Autodesk Inventor part; units mm, degrees
ref_plane "YZ Plane" through (0, 0, 0) normal (1, 0, 0) x (0, 1, 0)
ref_plane "XZ Plane" through (0, 0, 0) normal (0, 1, 0) x (-1, 0, 0)
ref_plane "XY Plane" through (0, 0, 0) normal (0, 0, 1) x (1, 0, 0)
sketch "Sketch1" plane through (0, 0, 0) normal (0, 1, 0) x (-1, 0, 0)
  line L0 (0, 0) -> (111.125, 0)
  line L1 (111.125, 0) -> (111.125, -88.9)
  line L2 (111.125, -88.9) -> (0, -88.9)
  line L3 (0, -88.9) -> (0, 0)
  dimension "d0" = 111.125
  dimension "d1" = 88.9
extrude "Extrusion1" add sketch "Sketch1" along normal blind 25.4
sketch "Sketch2" plane through (0, 25.4, 0) normal (0, 1, 0) x (1, 0, 0)
  line L0 (0, 88.9) -> (-111.125, 88.9)
  line L1 (-111.125, 0) -> (0, 0)
  line L2 (-27.305, 88.9) -> (-81.915, 88.9)
  line L3 (-81.915, 88.9) -> (-81.915, 0)
  line L4 (-81.915, 0) -> (-27.305, 0)
  line L5 (-27.305, 0) -> (-27.305, 88.9)
  line L6 (0, 0) -> (0, 88.9)
  dimension "d4" = 111.125
  dimension "d5" = 54.61
  dimension "d6" = 27.305
extrude "Extrusion2" cut sketch "Sketch2" against normal blind 3.175 contours L5 L1 L3 L0
sketch "Sketch4" plane through (-111.125, 0, 0) normal (0, 0, 1) x (1, 0, 0)
  line L0 (0, 0) -> (0, 25.4)
  line L1 (0, 19.05) -> (21.59, 25.4)
  line L2 (0, 25.4) -> (29.21, 25.4)
  point P0 (111.125, 0)
  dimension "d17" = 6.35
  dimension "d18" = 7.62
extrude "Extrusion4" cut sketch "Sketch4" against normal through all
fillet "Fillet2" radius 3.175 2 edges at (-111.125, 0, -44.45) (0, 25.4, -44.45)
properties part number "lift holder" material "PC/ABS Plastic"
Geometry check sheet. Reference: the model listing, model coordinates, mm. A direction names the side the tool comes from. Round coordinates to 2 decimals unless told otherwise and drop trailing zeros. Order: outer loops, then holes, each group sorted by start corner. A loop starts at its lowest first (then second) coordinate and runs counter-clockwise, first axis right, second up. Notation, with made-up numbers: M 16,82 L 66,82 A14 ccw 66,94 Z; hole C 13,63 d7. An arc over 180 degrees is marked long. Answer in a Markdown table with one row per item.
(1) Sectioned sample at A-A, the plane z = -17. Record the cut outline in (x, y) (3 decimals).
Responses:
| item | result |
|---|---|
| outline | M -111.125,3.175 A3.175 ccw -107.95,0 L 0,0 L 0,22.225 A3.175 ccw -3.175,25.4 L -27.305,25.4 L -27.305,22.225 L -81.915,22.225 L -81.915,25.4 L -89.535,25.4 L -111.125,19.05 Z |
(2) Go/stop test with flat-tipped pins: P1, Ø10, axis at x = -67, y = 8.5, coming from the +Z side; P2, Ø1, axis at y = 24, z = -29, coming from the +X side. Record where each tip stops, or that it passes through.
Responses:
| item | result |
|---|---|
| P1 | stops at z = 0 |
| P2 | stops at x = -0.27 |
(3) Tool access check on faces 1 (the face through (-56, 13, -88.9)), 2 (the face through (-55, 22.225, -45)). Record the directions out of +Z, -Z, +X, -X, +Y, -Y that give a thin tool (end or side, any length) a straight path to the whole face; none if there is none.
Responses:
| item | result |
|---|---|
| face 1 | -Z, +X, -X, +Y, -Y |
| face 2 | +Z, -Z, +Y |
(4) Draft check along X on faces 3 (the face through (-110.17, 0.905, -45.072)), 4 (the face through (-27.305, 24, -44)), 5 (the face through (-53, 0, -44)). Enter one of: released by +X, released by -X, zero draft, split by the parting line, or undercut.
Responses:
| item | result |
|---|---|
| face 3 | released by -X |
| face 4 | undercut |
| face 5 | zero draft |
(5) Scan lines: probe 1 along Y at (x, z) = (-52, -67.5) (3 decimals); probe 2 along X at (y, z) = (2.5, -28); probe 3 along Y at (x, z) = (-92, -67.5) (3 decimals). Record each from-to range of solid material in increasing order. Write a range as from..to.
Responses:
| item | result |
|---|---|
| probe 1 | y = 0..22.225 |
| probe 2 | x = -111.05..0 |
| probe 3 | y = 0..24.675 |
(6) Sectioned sample at B-B, the plane x = -29. Record the cut outline in (y, z) (3 decimals), and give its area (3 significant figures).
Responses:
| item | result |
|---|---|
| outline | M 0,-88.9 L 22.225,-88.9 L 22.225,0 L 0,0 Z |
| area | 1,980 mm² |
